from build123d import *

# Parameters (mm, degrees)
SKETCH1_R           = 25
BOSS_EXTRUDE1_DEPTH = 150
SKETCH2_R           = 2.5
BOSS_EXTRUDE2_DEPTH = 20
SKETCH3_W           = 1
SKETCH3_H           = 26.625756483
CUT_EXTRUDE1_DEPTH  = 174.637553542


with BuildPart() as part:
    # Sketch1 → Boss-Extrude1 (new body)
    with BuildSketch(Plane(origin=(0, 0, 0), x_dir=(1, 0, 0), z_dir=(0, 1, 0))):
        with Locations(Location((0, 0, 0), (0, 0, 270))):
            Circle(SKETCH1_R)
    extrude(amount=BOSS_EXTRUDE1_DEPTH)

    # Sketch2 → Boss-Extrude2 (add)
    with BuildSketch(Plane(origin=(0, 150, 0), x_dir=(1, 0, 0), z_dir=(0, 1, 0))):
        with Locations(Location((0, 0, 0), (0, 0, 270))):
            Circle(SKETCH2_R)
    extrude(amount=BOSS_EXTRUDE2_DEPTH)

    # Sketch3 → Cut-Extrude1 (cut, through all)
    with BuildSketch(Plane.XZ):
        with Locations((0, 15.674840511)):
            Rectangle(SKETCH3_W, SKETCH3_H)
    extrude(amount=-CUT_EXTRUDE1_DEPTH, mode=Mode.SUBTRACT)


solid = part.part
Verification items for the finished model (mm, model axes). A direction names the side the tool comes from. Coordinates: 2 decimals unless noted, no trailing zeros. Loops run counter-clockwise (first coordinate to the right, second up) from the corner with the lowest first, then second, coordinate; pieces in that order, holes last. Notation, with made-up numbers: (-33, 24.5) -> (26, 24.5) arc R24 cw to (26, 51.5) -> close; hole circle Ø1 at (-17, 25.5). An arc over 180 degrees is marked (long way). Answer as a JSON object with one key per item and string values. Group by question number.
Item 1: Sectioned sample at C-C on x = -15. Record the boundary of the cut face in (y, z), plus the area to 3 significant figures.
Item 2: Sectioned sample at D-D on y = 136.5. Record the boundary of the cut face in (x, z) (3 decimals), plus the area to 3 significant figures.
Item 3: Scan lines: probe 1 along Y at (x, z) = (-9.5, -20.5); probe 2 along X at (y, z) = (9, 22); probe 3 along Z at (x, y) = (11, 81). Record each from-to range of solid material in increasing order.
Item 4: Sectioned sample at A-A on z = 7. Record the boundary of the cut face in (x, y).
Item 5: Sectioned sample at B-B on z = 0. Record the boundary of the cut face in (x, y), plus the area to 3 significant figures.
Item 6: Mould release check, pull along X, two halves, no side actions. Record for faces 1 (the flat face through (0, 170, 0)), 2 (the cylindrical face through (1.092, 73.95, -24.976)), 3 (the flat face through (-0.5, 84, 14)), 4 (the flat face through (0.5, 84, 14)): +X half, -X half, draft (parallel to the pull), parting line (faces both ways), or undercut.
Item 7: Depth check by flat-ended pin: pin 1 (4 mm diameter, centred on x = 6, y = 70, fed in from -Z); pin 2 (12 mm diameter, centred on x = 14, z = -7.5, fed in from +Y); pin 3 (1.5 mm diameter, centred on y = 91, z = -12.5, fed in from +X). Enter the tip coordinate at first touch or a pass-through.
Item 8: Tool access check on faces 5 (the cylindrical face through (0.1, 159.9, -2.5)), 6 (the flat face through (0, 0, 0)). Record the directions out of +Z, -Z, +X, -X, +Y, -Y that give a thin tool (end or side, any length) a straight path to the whole face; none if there is none.
Evaluation:
{
 "1": {"outline": "(0, -20) -> (150, -20) -> (150, 20) -> (0, 20) -> close", "area": "6,000 mm²"},
 "2": {"outline": "(-0.5, 2.362) -> (-0.5, 24.995) arc R25 ccw (long way) to (0.5, 24.995) -> (0.5, 2.362) -> close", "area": "1,940 mm²"},
 "3": {"probe 1": "y = 0 to 150", "probe 2": "x = -11.87 to -0.5, 0.5 to 11.87", "probe 3": "z = -22.45 to 22.45"},
 "4": {"outline": "(-24, 0) -> (-0.5, 0) -> (-0.5, 150) -> (-24, 150) -> close; (0.5, 0) -> (24, 0) -> (24, 150) -> (0.5, 150) -> close"},
 "5": {"outline": "(-25, 0) -> (25, 0) -> (25, 150) -> (2.5, 150) -> (2.5, 170) -> (-2.5, 170) -> (-2.5, 150) -> (-25, 150) -> close", "area": "7,600 mm²"},
 "6": {"face 1": "draft", "face 2": "parting line", "face 3": "undercut", "face 4": "undercut"},
 "7": {"pin 1": "stops at z = -24.68", "pin 2": "stops at y = 150", "pin 3": "stops at x = 22.07"},
 "8": {"face 5": "+Y", "face 6": "+Z, -Z, +X, -X, -Y"}
}
